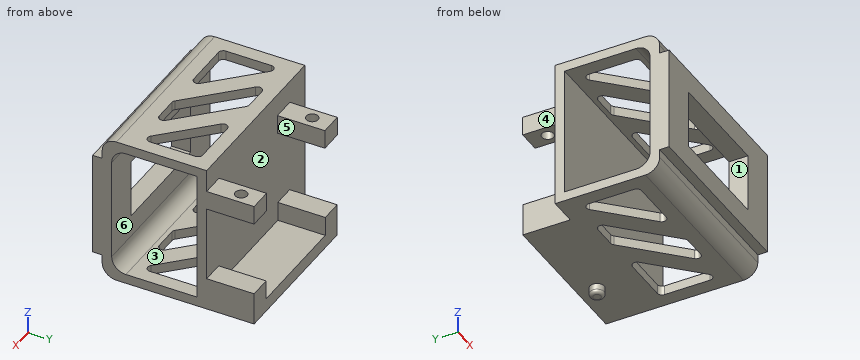
from build123d import *

# Parameters (mm, degrees)
SKETCH1_W           = 38
SKETCH1_H           = 22
SKETCH1_W_2         = 23
SKETCH1_H_2         = 12.3
BOSS_EXTRUDE1_DEPTH = 4
BOSS_EXTRUDE2_DEPTH = 38
FILLET1_R           = 3
CUT_EXTRUDE5_DEPTH  = 44.923228479
FILLET3_R           = 1
MIRROR1_START       = 13.75
MIRROR1_DEPTH       = 2
SKETCH10_W          = 4.8
SKETCH10_H          = 4
BOSS_EXTRUDE4_DEPTH = 10
SKETCH11_R          = 1.25
CUT_EXTRUDE6_DEPTH  = 48.25
BOSS_EXTRUDE5_DEPTH = 10
BOSS_EXTRUDE6_START = -15.75
SKETCH14_R          = 1.5
BOSS_EXTRUDE6_DEPTH = 2
FILLET4_R           = 0.7


# Read off the part's stored shape, not the designer's step: Mirror1
with BuildPart() as part:
    # Sketch1 → Boss-Extrude1 (new body)
    with BuildSketch(Plane(origin=(0, 0, 0), x_dir=(1, 0, 0), z_dir=(0, 1, 0))):
        Rectangle(SKETCH1_W, SKETCH1_H)
        Rectangle(SKETCH1_W_2, SKETCH1_H_2, mode=Mode.SUBTRACT)
    extrude(amount=BOSS_EXTRUDE1_DEPTH)

    # Sketch2 → Boss-Extrude2 (add)
    with BuildSketch(Plane.ZY.offset(19)):
        Polygon((-11, 2), (-15.75, 2), (-15.75, 22), (-15.75, 24), (15.75, 24), (15.75, 22), (15.75, 2), (11, 2), (11, 4), (13.75, 4), (13.75, 22), (-13.75, 22), (-13.75, 4), (-11, 4), align=None)
    extrude(amount=-BOSS_EXTRUDE2_DEPTH)

    # Fillet1
    fillet1_edges = [part.edges().sort_by_distance(p)[0] for p in [
        (0, 2, -15.75),
        (0, 2, 15.75),
        (0, 4, 13.75),
        (0, 4, -13.75),
    ]]
    fillet(fillet1_edges, radius=FILLET1_R)

    # Sketch8 → Cut-Extrude5 (cut, through all)
    with BuildSketch(Plane(origin=(0, 0, -15.75), x_dir=(-1, 0, 0), z_dir=(0, 0, -1))):
        Polygon((-16, 8), (-16, 21), (-3, 21), align=None)
        Polygon((3, 8), (16, 21), (16, 8), align=None)
        Polygon((-10.343145751, 8), (-2.656854249, 8), (10.343145751, 21), (2.656854249, 21), align=None)
    extrude(amount=-CUT_EXTRUDE5_DEPTH, mode=Mode.SUBTRACT)

    # Fillet3
    fillet3_edges = [part.edges().sort_by_distance(p)[0] for p in [
        (-16, 8, -14.75),
        (-3, 8, -14.75),
        (-16, 21, -14.75),
        (10.343145751, 8, -14.75),
        (-2.656854249, 21, -14.75),
        (-10.343145751, 21, -14.75),
        (2.656854249, 8, -14.75),
        (3, 21, -14.75),
        (16, 8, -14.75),
        (16, 21, -14.75),
    ]]
    fillet(fillet3_edges, radius=FILLET3_R)

    # Mirror1 outline → Mirror1 (add)
    with BuildSketch(Plane.XY.offset(MIRROR1_START)):
        with BuildLine():
            ThreePointArc((15, 21), (15.707106781, 20.707106781), (16, 20))
            Line((16, 20), (16, 21))
            Line((16, 21), (15, 21))
        make_face()
        with BuildLine():
            Line((16, 8), (16, 10.414213562))
            ThreePointArc((16, 10.414213562), (15.382683432, 9.49033403), (14.292893219, 9.707106781))
            Line((14.292893219, 9.707106781), (16, 8))
        make_face()
        with BuildLine():
            ThreePointArc((4.707106781, 19.292893219), (4.49033403, 20.382683432), (5.414213562, 21))
            Line((5.414213562, 21), (3, 21))
            Line((3, 21), (4.707106781, 19.292893219))
        make_face()
        with BuildLine():
            ThreePointArc((-15, 8), (-15.707106781, 8.292893219), (-16, 9))
            Line((-16, 9), (-16, 8))
            Line((-16, 8), (-15, 8))
        make_face()
        with BuildLine():
            Line((-16, 21), (-16, 18.585786438))
            ThreePointArc((-16, 18.585786438), (-15.382683432, 19.50966597), (-14.292893219, 19.292893219))
            Line((-14.292893219, 19.292893219), (-16, 21))
        make_face()
        with BuildLine():
            ThreePointArc((-4.707106781, 9.707106781), (-4.49033403, 8.617316568), (-5.414213562, 8))
            Line((-5.414213562, 8), (-3, 8))
            Line((-3, 8), (-4.707106781, 9.707106781))
        make_face()
        with BuildLine():
            ThreePointArc((8.636038969, 9.707106781), (8.852811721, 8.617316567), (7.928932188, 8))
            Line((7.928932188, 8), (10.343145751, 8))
            Line((10.343145751, 8), (8.636038969, 9.707106781))
        make_face()
        with BuildLine():
            Line((2.656854249, 8), (3.071067812, 8))
            ThreePointArc((3.071067812, 8), (2.68838438, 8.076120467), (2.363961031, 8.292893219))
            Line((2.363961031, 8.292893219), (2.656854249, 8))
        make_face()
        with BuildLine():
            ThreePointArc((-3.071067812, 21), (-2.68838438, 20.923879533), (-2.363961031, 20.707106781))
            Line((-2.363961031, 20.707106781), (-2.656854249, 21))
            Line((-2.656854249, 21), (-3.071067812, 21))
        make_face()
        with BuildLine():
            Line((-10.343145751, 21), (-8.636038969, 19.292893219))
            ThreePointArc((-8.636038969, 19.292893219), (-8.852811721, 20.382683433), (-7.928932188, 21))
            Line((-7.928932188, 21), (-10.343145751, 21))
        make_face()
    extrude(amount=MIRROR1_DEPTH)

    # Sketch10 → Boss-Extrude4 (add)
    with BuildSketch(Plane(origin=(0, 24, 0), x_dir=(1, 0, 0), z_dir=(0, 1, 0))):
        with Locations((-10.8, -9)):
            Rectangle(SKETCH10_W, SKETCH10_H)
        with Locations((16.6, -9)):
            Rectangle(SKETCH10_W, SKETCH10_H)
    extrude(amount=BOSS_EXTRUDE4_DEPTH)

    # Sketch11 → Cut-Extrude6 (cut, through all)
    with BuildSketch(Plane.XY.offset(11)):
        with Locations((16.65, 30)):
            Circle(SKETCH11_R)
        with Locations((-10.85, 30)):
            Circle(SKETCH11_R)
    extrude(amount=-CUT_EXTRUDE6_DEPTH, mode=Mode.SUBTRACT)

    # Sketch12 → Boss-Extrude5 (add)
    with BuildSketch(Plane(origin=(0, 24, 0), x_dir=(1, 0, 0), z_dir=(0, 1, 0))):
        Polygon((-8.55, 8.870549132), (-13.15, 8.870549132), (-13.15, 15.75), (19, 15.75), (19, 8.870549132), (14.35, 8.870549132), (14.35, 12.95), (-8.55, 12.95), align=None)
    extrude(amount=BOSS_EXTRUDE5_DEPTH)

    # Sketch14 → Boss-Extrude6 (add)
    with BuildSketch(Plane.XY.offset(BOSS_EXTRUDE6_START)):
        with Locations(Location((8.25, 30, 0), (0, 0, 180))):
            Circle(SKETCH14_R)
    extrude(amount=-BOSS_EXTRUDE6_DEPTH)

    # Fillet4
    fillet4_edges = [part.edges().sort_by_distance(p)[0] for p in [
        (9.75, 30, -17.75),
    ]]
    fillet(fillet4_edges, radius=FILLET4_R)


solid = part.part
Work out the finished part from the listing and answer in its coordinate system (mm). Face numbers are marked on the shaded views. A direction names the side the tool comes from. Round coordinates to 2 decimals unless told otherwise and drop trailing zeros. Loops run counter-clockwise (first coordinate to the right, second up) from the corner with the lowest first, then second, coordinate; pieces in that order, holes last. Notation, with made-up numbers: M 27.5,-10.75 L 74.5,-10.75 A23 cw 74.5,17.25 Z; hole C 69,86.5 d11. An arc over 180 degrees is marked long. One line per question, with ' | ' between items. Start each with the question number.
(1) A cutting plane is placed at A-A on x = 16.65. Write down the section's boundary in (y, z).
(2) Flat-ended cylindrical pins translate along their axes: pin 1 Ø3 at (x, z) = (-9, -6) entering from +Y; pin 2 Ø2 at (x, z) = (-5.5, -14.5) entering from -Y; pin 3 Ø12 at (x, y) = (0.5, 11.5) entering from -Z. Find the tip coordinate at first contact, or state that the pin passes through.
(3) Find the intervals of material crossed by line 1 (Y direction, x = -10.85, z = 9.9); line 2 (Y direction, x = -10, z = 8); line 3 (Z direction, x = -6.5, y = 15), in increasing order.
(4) For a pull along X with two mould halves and no side action, classify the marked faces 4, 5 and 6 as released by +X, released by -X, zero draft, split by the parting line, or undercut.
(5) A cutting plane is placed at D-D on y = 3. Write down the section's boundary in (x, z), plus the area to 3 significant figures.
(6) A cutting plane is placed at B-B on y = 30. Give the number of separate pieces and of enclosed holes in the cut face, plus the area to 3 significant figures.
(7) A tool of negligible diameter and unlimited length cuts with its end or side. For the marked faces 1, 2 and 3, from which of +Z, -Z, +X, -X, +Y, -Y can it reach the whole face along a straight path? Write none if from no direction.
(8) A cutting plane is placed at C-C on z = -4.5. Write down the section's boundary in (x, y), plus the area to 3 significant figures.
Geometry check:
1) outline: M 0,-11 L 2,-11 L 2,-12.75 A3 ccw 5,-15.75 L 34,-15.75 L 34,-8.87 L 24,-8.87 L 24,7 L 28.75,7 L 28.75,11 L 24,11 L 24,15.75 L 5,15.75 A3 ccw 2,12.75 L 2,11 L 0,11 Z; M 31.25,7 L 34,7 L 34,11 L 31.25,11 Z; hole M 4,-10.75 A3 ccw 7,-13.75 L 22,-13.75 L 22,13.75 L 7,13.75 A3 ccw 4,10.75 Z
2) pin 1: stops at y = 24 | pin 2: stops at y = 2.1 | pin 3: stops at z = -15.75
3) line 1: y = 0 to 4, 22 to 28.75, 31.25 to 34 | line 2: y = 0 to 4, 22 to 29.08, 30.92 to 34 | line 3: z = -15.75 to -13.75, 13.75 to 15.75
4) face 4: released by -X | face 5: undercut | face 6: zero draft
5) outline: M -19,-14.99 L 19,-14.99 L 19,14.99 L -19,14.99 Z; hole M -11.5,-6.15 L 11.5,-6.15 L 11.5,6.15 L -11.5,6.15 Z | area: 856 mm²
6) separate pieces: 5 | enclosed holes: 0 | area: 152 mm²
7) face 1: -Y | face 2: +Y | face 3: +X, -X
8) outline: M -19,0 L -11.5,0 L -11.5,4 L -19,4 Z; M -19,22 L 19,22 L 19,24 L -19,24 Z; M 11.5,0 L 19,0 L 19,4 L 11.5,4 Z | area: 136 mm²
